Can you work these out from the model? Positions are in its coordinate system, mm. Face numbers are marked on the shaded views. A direction names the side the tool comes from. Give positions to 0.01 mm unless a question says otherwise; leave off trailing zeros. Loops run counter-clockwise (first coordinate to the right, second up) from the corner with the lowest first, then second, coordinate; pieces in that order, holes last. Notation, with made-up numbers: M 35,-10 L 53,-10 A30 cw 53,16 Z; hole C 12.25,-25 d2. An arc over 180 degrees is marked long. Answer as a JSON object with one key per item and string values.
```python
from build123d import *

# Parameters (mm, degrees)
SKETCH1_W               = 60
SKETCH1_H               = 20
BOSS_EXTRUDE1_DEPTH     = 30
CUT_EXTRUDE1_DEPTH      = 47.904157598
CUT_EXTRUDE2_START      = -4
CUT_EXTRUDE2_DEPTH      = 43.904157598
CUT_EXTRUDE3_DEPTH      = 68.823299831
CUT_EXTRUDE3_DEPTH_BACK = 68.823299831
SKETCH5_R               = 1.75
CUT_EXTRUDE4_DEPTH      = 44.27017093
CUT_EXTRUDE5_DEPTH      = 5
FILLET1_R               = 5


with BuildPart() as part:
    # Sketch1 → Boss-Extrude1 (new body)
    with BuildSketch(Plane.XY):
        Rectangle(SKETCH1_W, SKETCH1_H)
    extrude(amount=BOSS_EXTRUDE1_DEPTH)

    # Sketch2 → Cut-Extrude1 (cut, through all)
    with BuildSketch(Plane(origin=(0, 10, 0), x_dir=(1, 0, 0), z_dir=(0, 1, 0))):
        Polygon((-30, -30), (30, -30), (-30, -22.5), align=None)
    extrude(amount=-CUT_EXTRUDE1_DEPTH, mode=Mode.SUBTRACT)

    # Sketch3 → Cut-Extrude2 (cut, through all)
    with BuildSketch(Plane(origin=(0, 10, 0), x_dir=(1, 0, 0), z_dir=(0, 1, 0)).offset(CUT_EXTRUDE2_START)):
        Polygon((-25, 0), (25, 0), (25, -24.336088907), (-25, -18.086088907), align=None)
    extrude(amount=-CUT_EXTRUDE2_DEPTH, mode=Mode.SUBTRACT)

    # Sketch4 → Cut-Extrude3 (cut, two sides: drawn at the far end of the back side and taken through both)
    with BuildSketch(Plane.ZY.offset(30).offset(-CUT_EXTRUDE3_DEPTH_BACK)):
        Polygon((4, 1.75), (0, 1.75), (0, -1.75), (4, -1.75), (4, -2.85), (7, -2.85), (7, -1.75), (10, -1.75), (10, 1.75), (7, 1.75), (7, 2.85), (4, 2.85), align=None)
    extrude(amount=CUT_EXTRUDE3_DEPTH + CUT_EXTRUDE3_DEPTH_BACK, mode=Mode.SUBTRACT)

    # Sketch5 → Cut-Extrude4 (cut, through all)
    with BuildSketch(Plane(origin=(-3.230769231, 0, 25.846153846), x_dir=(0.9922778767136677, 0, 0.12403473458920845), z_dir=(-0.12403473458920845, 0, 0.9922778767136677))):
        with Locations((21.755911783, 0)):
            Circle(SKETCH5_R)
        with Locations((-15.244088217, 0)):
            Circle(SKETCH5_R)
    extrude(amount=-CUT_EXTRUDE4_DEPTH, mode=Mode.SUBTRACT)

    # Sketch6 → Cut-Extrude5 (cut)
    with BuildSketch(Plane(origin=(-3.230769231, 0, 25.846153846), x_dir=(0.9922778767136677, 0, 0.12403473458920845), z_dir=(-0.12403473458920845, 0, 0.9922778767136677))):
        with BuildLine():
            Line((-13.494088217, 5), (-13.494088217, -5))
            ThreePointArc((-13.494088217, -5), (-15.244088217, -6.75), (-16.994088217, -5))
            Line((-16.994088217, -5), (-16.994088217, 5))
            ThreePointArc((-16.994088217, 5), (-15.244088217, 6.75), (-13.494088217, 5))
        make_face()
        with BuildLine():
            Line((20.005911783, 5), (20.005911783, -5))
            ThreePointArc((20.005911783, -5), (21.755911783, -6.75), (23.505911783, -5))
            Line((23.505911783, -5), (23.505911783, 5))
            ThreePointArc((23.505911783, 5), (21.755911783, 6.75), (20.005911783, 5))
        make_face()
    extrude(amount=-CUT_EXTRUDE5_DEPTH, mode=Mode.SUBTRACT)

    # Fillet1
    fillet1_edges = [part.edges().sort_by_distance(p)[0] for p in [
        (-30, 0, 22.5),
        (30, 0, 30),
    ]]
    fillet(fillet1_edges, radius=FILLET1_R)


solid = part.part
```
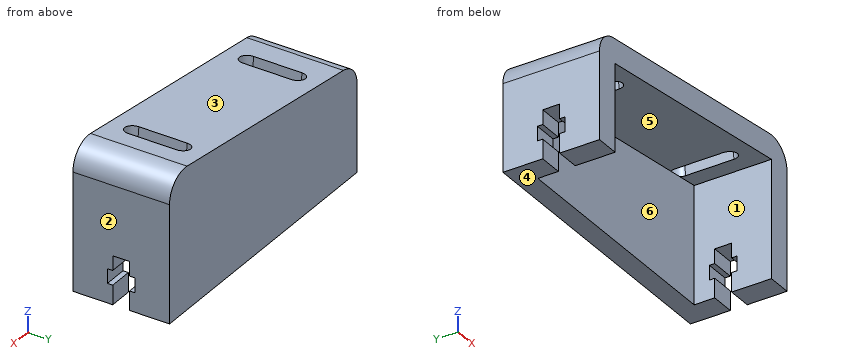
1) Suppose I cut it at D-D, the plane x = 4. Write out the boundary of the cut face in (y, z).
Answer list:
{"outline": "M -10,21.71 L 6,21.71 L 6,0 L 10,0 L 10,26.75 L -10,26.75 Z"}
2) Will these pins go through, and if not, where does the flat tip stop? pin 1 Ø0.9 at (x, y) = (-27, 2.5) entering from +Z; pin 2 Ø3 at (x, z) = (9, 21) entering from -Y; pin 3 Ø1 at (x, z) = (-14.5, 11.5) entering from -Y; pin 4 Ø1.5 at (x, y) = (-22, -1) entering from +Z.
Answer list:
{"pin 1": "z = 22.84", "pin 2": "y = -10", "pin 3": "y = 6", "pin 4": "z = 23.59"}
3) Suppose I cut it at B-B, the plane y = -8.25. Write out the boundary of the cut face in (x, z), and give its area (3 significant figures).
Answer list:
{"outline": "M -30,0 L -25,0 L -25,18.09 L 25,24.34 L 25,0 L 30,0 L 30,24.34 A5 ccw 24.38,29.3 L -25.62,23.05 A5 ccw -30,18.09 Z", "area": "503 mm^2"}
4) For the marked faces 1 and 2, which set-ups out of +Z, -Z, +X, -X, +Y, -Y let a thin tool reach every point of the face, with its end or its side?
Answer list:
{"face 1": "-Z, -Y", "face 2": "+Z, -Z, +X, +Y, -Y"}
5) Please list where these lines run through material, in increasing order: line 1 along X through (y, z) = (-6.25, 10.5); line 2 along Y through (x, z) = (-22.5, 4.25); line 3 along Z through (x, y) = (-9, 9.25) (3 decimals). Write a range as from..to.
Answer list:
{"line 1": "-30..-25, 25..30", "line 2": "6..10", "line 3": "0..25.125"}
6) If we mould it in two halves opening along X, with no side actions, what happens to the marked faces 3, 4, 5 and 6? For each: +X half, -X half, draft (parallel to the pull), parting line (faces both ways), or undercut.
Answer list:
{"face 3": "-X half", "face 4": "draft", "face 5": "undercut", "face 6": "undercut"}
7) Suppose I cut it at C-C, the plane z = 12. Write out the boundary of the cut face in (x, y), and give its area (3 significant figures).
Answer list:
{"outline": "M -30,-10 L -25,-10 L -25,6 L 25,6 L 25,-10 L 30,-10 L 30,10 L -30,10 Z", "area": "400 mm^2"}
8) Suppose I cut it at A-A, the plane z = 5. Write out the boundary of the cut face in (x, y), and give its area (3 significant figures).
Answer list:
{"outline": "M -30,-10 L -25,-10 L -25,-2.85 L -30,-2.85 Z; M -30,2.85 L -25,2.85 L -25,6 L 25,6 L 25,2.85 L 30,2.85 L 30,10 L -30,10 Z; M 25,-10 L 30,-10 L 30,-2.85 L 25,-2.85 Z", "area": "343 mm^2"}
